from build123d import *

# Parameters (mm, degrees)
SKETCH_W             = 20
SKETCH_H             = 20
PAD_DEPTH            = 306
SKETCH001_R          = 2.5
POCKET_DEPTH         = 306.001
POCKET001_DEPTH      = 306.001
BODY_PLACEMENT_ANGLE = 90


with BuildPart() as part:
    # Sketch → Pad (new body)
    with BuildSketch(Plane.XY):
        Rectangle(SKETCH_W, SKETCH_H)
    extrude(amount=PAD_DEPTH)

    # Sketch001 (on Face6 of Pad) → Pocket (cut, through all)
    with BuildSketch(Plane.XY.offset(306)):
        Circle(SKETCH001_R)
        Polygon((-3.1, 10), (3.1, 10), (3.1, 8), (6.232233, 8), (2.132233, 3.9), (-2.132233, 3.9), (-6.232233, 8), (-3.1, 8), align=None)
        Polygon((-3.1, -8), (-6.232233, -8), (-2.132233, -3.9), (2.132233, -3.9), (6.232233, -8), (3.1, -8), (3.1, -10), (-3.1, -10), align=None)
    extrude(amount=-POCKET_DEPTH, mode=Mode.SUBTRACT)

    # Sketch002 (on Face2 of Pocket) → Pocket001 (cut, through all)
    with BuildSketch(Plane(origin=(0, 0, 0), x_dir=(1, 0, 0), z_dir=(0, 0, -1))):
        Polygon((-10, -3.1), (-8, -3.1), (-8, -6.232233), (-3.9, -2.132233), (-3.9, 2.132233), (-8, 6.232233), (-8, 3.1), (-10, 3.1), align=None)
        Polygon((3.9, -2.132233), (3.9, 2.132233), (8, 6.232233), (8, 3.1), (10, 3.1), (10, -3.1), (8, -3.1), (8, -6.232233), align=None)
    extrude(amount=-POCKET001_DEPTH, mode=Mode.SUBTRACT)


with BuildPart() as part_1:
    # Body placement: moved
    add(part.part.moved(Location((-76, 0, 0))).rotate(Axis((-76, 0, 0), (1, 0, 0)), BODY_PLACEMENT_ANGLE))


solid = part_1.part
CAD build for the part. Positions are in the model's coordinates, mm. Round coordinates to 2 decimals unless told otherwise and drop trailing zeros. Use a Markdown table: item, result. Add a question column.
1. Pull direction Z, two halves, no side cores. Call faces 1 (the face through (-78.5, -155.1, 0.1)), 2 (the face through (-69, -151, 10)), 3 (the face through (-86, -151, 7)): released by +Z, released by -Z, zero draft, split by the parting line, or undercut.
2. Drill centre lines: probe 1 along X at (y, z) = (-69, 9.25); probe 2 along Z at (x, y) = (-76, -69); probe 3 along Z at (x, y) = (-67.25, -83). Where is each one in solid material? Low to high.
3. Flat gauge pins, fed straight in: P1, Ø4.5, axis at x = -76, z = 0, coming from the -Y side; P2, Ø2, axis at y = -128, z = 1, coming from the -X side; P3, Ø1.3, axis at y = -151.5, z = 0, coming from the +X side; P4, Ø1.3, axis at x = -77, y = -154.5, coming from the -Z side. Where does each tip first touch, or does it go through?
Reply:
| question | item | result |
|---|---|---|
| 1 | face 1 | undercut |
| 1 | face 2 | released by +Z |
| 1 | face 3 | zero draft |
| 2 | probe 1 | x = -86 to -79.1, -72.9 to -66 |
| 2 | probe 2 | z = -3.9 to -2.5, 2.5 to 3.9 |
| 2 | probe 3 | z = -10 to -3.1, 3.1 to 10 |
| 3 | P1 | passes through |
| 3 | P2 | stops at x = -79.9 |
| 3 | P3 | stops at x = -72.1 |
| 3 | P4 | stops at z = -3.9 |
